from build123d import *

# Parameters (mm, degrees)
SKETCH1_R               = 76.2
BOSS_EXTRUDE1_DEPTH     = 3.175
CUT_EXTRUDE1_REACH      = 109.81
SKETCH2_R               = 7
CUT_EXTRUDE3_DEPTH      = 108.809835474
CUT_EXTRUDE3_DEPTH_BACK = 108.809835474
SKETCH4_R               = 3.175
M4_CLEARANCE_HOLE1_D    = 4.5
CUT_EXTRUDE4_REACH      = 109.81
SKETCH8_R               = 1.89865
CUT_EXTRUDE5_REACH      = 109.81
SKETCH9_R               = 2.032


with BuildPart() as part:
    # Sketch1 → Boss-Extrude1 (new body)
    with BuildSketch(Plane(origin=(0, 0, 0), x_dir=(1, 0, 0), z_dir=(0, 1, 0))):
        with Locations(Location((0, 0, 0), (0, 0, 270))):
            Circle(SKETCH1_R)
    extrude(amount=BOSS_EXTRUDE1_DEPTH)

    # Sketch2 → Cut-Extrude1 (cut, up to next)
    with BuildSketch(Plane(origin=(0, 3.175, 0), x_dir=(1, 0, 0), z_dir=(0, 1, 0)), mode=Mode.PRIVATE) as cut_extrude1_sk1:
        with Locations(Location((0, 0, 0), (0, 0, 270))):
            Circle(SKETCH2_R)
    cut_extrude1_tool1 = extrude(cut_extrude1_sk1.sketch, amount=-CUT_EXTRUDE1_REACH, mode=Mode.PRIVATE) & part.part
    add(cut_extrude1_tool1.solids().sort_by_distance((0, 3.175, 0))[0], mode=Mode.SUBTRACT)

    # Sketch4 → Cut-Extrude3 (cut, two sides: drawn at the far end of the back side and taken through both)
    with BuildSketch(Plane(origin=(0, 3.175, 0), x_dir=(1, 0, 0), z_dir=(0, 1, 0)).offset(-CUT_EXTRUDE3_DEPTH_BACK)):
        with Locations(Location((-22.225, 0, 0), (0, 0, 270))):
            Circle(SKETCH4_R)
        with Locations(Location((22.225, 0, 0), (0, 0, 270))):
            Circle(SKETCH4_R)
    extrude(amount=CUT_EXTRUDE3_DEPTH + CUT_EXTRUDE3_DEPTH_BACK, mode=Mode.SUBTRACT)

    # M4 Clearance Hole1 (through all)
    with Locations(Plane(origin=(0, 3.175, 0), x_dir=(1, 0, 0), z_dir=(0, 1, 0))):
        with Locations((-8, 8), (8, 8), (8, -8), (-8, -8)):
            Hole(M4_CLEARANCE_HOLE1_D / 2)

    # Sketch8 → Cut-Extrude4 (cut, up to next)
    with BuildSketch(Plane(origin=(0, 3.175, 0), x_dir=(1, 0, 0), z_dir=(0, 1, 0)), mode=Mode.PRIVATE) as cut_extrude4_sk1:
        with Locations(Location((19.05, 38.1, 0), (0, 0, 270))):
            Circle(SKETCH8_R)
    cut_extrude4_tool1 = extrude(cut_extrude4_sk1.sketch, amount=-CUT_EXTRUDE4_REACH, mode=Mode.PRIVATE) & part.part
    # Sketch8 → Cut-Extrude4 (cut, up to next)
    with BuildSketch(Plane(origin=(0, 3.175, 0), x_dir=(1, 0, 0), z_dir=(0, 1, 0)), mode=Mode.PRIVATE) as cut_extrude4_sk2:
        with Locations(Location((-19.05, 38.1, 0), (0, 0, 270))):
            Circle(SKETCH8_R)
    cut_extrude4_tool2 = extrude(cut_extrude4_sk2.sketch, amount=-CUT_EXTRUDE4_REACH, mode=Mode.PRIVATE) & part.part
    add(cut_extrude4_tool1.solids().sort_by_distance((19.05, 3.175, -38.1))[0], mode=Mode.SUBTRACT)
    add(cut_extrude4_tool2.solids().sort_by_distance((-19.05, 3.175, -38.1))[0], mode=Mode.SUBTRACT)

    # Sketch9 → Cut-Extrude5 (cut, up to next)
    with BuildSketch(Plane.XZ, mode=Mode.PRIVATE) as cut_extrude5_sk1:
        with Locations(Location((-8, 22.86, 0), (0, 0, 270))):
            Circle(SKETCH9_R)
    cut_extrude5_tool1 = extrude(cut_extrude5_sk1.sketch, amount=-CUT_EXTRUDE5_REACH, mode=Mode.PRIVATE) & part.part
    # Sketch9 → Cut-Extrude5 (cut, up to next)
    with BuildSketch(Plane.XZ, mode=Mode.PRIVATE) as cut_extrude5_sk2:
        with Locations(Location((-8, 66.04, 0), (0, 0, 270))):
            Circle(SKETCH9_R)
    cut_extrude5_tool2 = extrude(cut_extrude5_sk2.sketch, amount=-CUT_EXTRUDE5_REACH, mode=Mode.PRIVATE) & part.part
    add(cut_extrude5_tool1.solids().sort_by_distance((-8, 0, 22.86))[0], mode=Mode.SUBTRACT)
    add(cut_extrude5_tool2.solids().sort_by_distance((-8, 0, 66.04))[0], mode=Mode.SUBTRACT)


solid = part.part
Geometry check sheet. Reference: the model listing, model coordinates, mm. Give positions to 0.01 mm unless a question says otherwise; leave off trailing zeros. Order: outer loops, then holes, each group sorted by start corner. A loop starts at its lowest first (then second) coordinate and runs counter-clockwise, first axis right, second up.
1. Sectioned sample at C-C (y = 0.65). State how many separate pieces and enclosed holes the cut face has, then the cut area to 3 significant figures.
Completed:
separate pieces: 1
enclosed holes: 11
area: 17,900 mm2
2. Depth check by flat-ended pin: pin 1 (3.5 mm diameter, centred on x = -8, z = 22.86, fed in from +Y); pin 2 (1.5 mm diameter, centred on x = -58, y = 2, fed in from +Z); pin 3 (1 mm diameter, centred on y = 1.5, z = 21, fed in from +X). Enter the tip coordinate at first touch or a pass-through.
Completed:
pin 1: passes through
pin 2: stops at z = 50.29
pin 3: stops at x = 73.39
3. Draft check along X on faces 1 (the face through (-46.367, 1.565, -60.47)), 2 (the face through (1, 0, 16)), 3 (the face through (-6.34, 1.57, -9.52)). Enter one of: pulls with the +X half, pulls with the -X half, needs draft (parallel to the pull), parting line crosses it, or undercut.
Completed:
face 1: parting line crosses it
face 2: needs draft
face 3: undercut
4. Sectioned sample at D-D (z = 22.86). Record the boundary of the cut face in (x, y) (3 decimals), then the cut area to 3 significant figures.
Completed:
outline: (-72.69, 0) - (-10.032, 0) - (-10.032, 3.175) - (-72.69, 3.175) - close; (-5.968, 0) - (72.69, 0) - (72.69, 3.175) - (-5.968, 3.175) - close
area: 449 mm2
5. Scan lines: line 1 (X direction, y = 1.4, z = 0); line 2 (Z direction, x = 8, y = 2.4). Record each from-to range of solid material in increasing order.
Completed:
line 1: x = -76.2 to -25.4, -19.05 to -7, 7 to 19.05, 25.4 to 76.2
line 2: z = -75.78 to -10.25, -5.75 to 5.75, 10.25 to 75.78
6. Sectioned sample at B-B (z = 0). Record the boundary of the cut face in (x, y) (3 decimals).
Completed:
outline: (-76.2, 0) - (-25.4, 0) - (-25.4, 3.175) - (-76.2, 3.175) - close; (-19.05, 0) - (-7, 0) - (-7, 3.175) - (-19.05, 3.175) - close; (7, 0) - (19.05, 0) - (19.05, 3.175) - (7, 3.175) - close; (25.4, 0) - (76.2, 0) - (76.2, 3.175) - (25.4, 3.175) - close
7. Sectioned sample at A-A (x = 0). Record the boundary of the cut face in (y, z) (3 decimals).
Completed:
outline: (0, -76.2) - (3.175, -76.2) - (3.175, -7) - (0, -7) - close; (0, 7) - (3.175, 7) - (3.175, 76.2) - (0, 76.2) - close
